Build history of the part. All positions in model axes, mm. A direction names the side the tool comes from. Round coordinates to 2 decimals unless told otherwise and drop trailing zeros. Loops run counter-clockwise (first coordinate to the right, second up) from the corner with the lowest first, then second, coordinate; pieces in that order, holes last. Notation, with made-up numbers: (-22.75, 24.25) -> (12.25, 24.25) arc R30 ccw to (12.25, 55.25) -> close; hole circle Ø9 at (47.25, 5). An arc over 180 degrees is marked (long way). Put each result on its own line as item: value. Start each with the question number.
Item 1: Cut at A-A, the plane x = 7.5. Count the separate pieces of the cut face and the enclosed holes in it, plus the area to 3 significant figures.
Item 2: Cut at D-D, the plane y = -10. List the corners of the cut face in (x, z), plus the area to 3 significant figures.
Item 3: Cut at C-C, the plane z = 26. List the corners of the cut face in (x, y).
Item 4: Pull direction Z, two halves, no side cores. Call faces 1 (the flat face through (15, -5, 27.5)), 2 (the flat face through (23, -23, 5)), 3 (the cylindrical face through (0.57, -39.4, 17.74)), 4 (the flat face through (3, -7.349, 29)): +Z half, -Z half, draft (parallel to the pull), parting line (faces both ways), or undercut.
Item 5: Flat gauge pins, fed straight in: pin 1 Ø5.5 at (x, y) = (22.5, -10) entering from +Z; pin 2 Ø3 at (x, y) = (7.5, -25) entering from -Z. Where does each tip first touch, or does it go through?
Item 6: Cut at B-B, the plane y = -5. List the corners of the cut face in (x, z).
Item 7: Drill centre lines: probe 1 along Y at (x, z) = (11, 28.5); probe 2 along Y at (x, z) = (22.5, 3.85); probe 3 along Z at (x, y) = (27.5, -5.5). Where is each one in solid material? Low to high. Write a range as [from, to].
Item 8: Tool access for faces 5 (the cylindrical face through (4.881, -12.008, 20.21)), 6 (the cylindrical face through (0.57, -0.6, 17.74)), 7 (the flat face through (15, -5, 30)): list every direction of +Z, -Z, +X, -X, +Y, -Y with a clear straight run to the whole face (end or side of a thin tool).
```python
from build123d import *

# Parameters (mm, degrees)
F0_W      = 30
F0_H      = 40
F1_DEPTH  = 35
F2_R      = 3.3
F3_DEPTH  = 30
F4_W      = 5
F4_H      = 2.5
F5_DEPTH  = 30.001
F6_R      = 1.65
F7_DEPTH  = 5.001
F8_R      = 1.65
F9_DEPTH  = 5.001
F10_R     = 1.65
F11_DEPTH = 5.001
F12_R     = 1.65
F13_DEPTH = 5.001
F14_R     = 2


with BuildPart() as f1:
    # F0 (on Top) → F1 (new body)
    with BuildSketch(Plane.XY):
        with Locations((15, -20)):
            Rectangle(F0_W, F0_H)
    extrude(amount=F1_DEPTH)

    # F2 (on face) → F3 (cut)
    with BuildSketch(Plane.XY.offset(35)):
        with Locations((7.5, -10)):
            Circle(F2_R)
        with Locations((22.5, -10)):
            Circle(F2_R)
        with Locations((7.5, -25)):
            Circle(F2_R)
        with Locations((22.5, -25)):
            Circle(F2_R)
    extrude(amount=-F3_DEPTH, mode=Mode.SUBTRACT)

    # F4 (on face) → F5 (cut, through all)
    with BuildSketch(Plane(origin=(0, 0, 0), x_dir=(0, -1, 0), z_dir=(-1, 0, 0))):
        with Locations((4.849052, 28.75)):
            Rectangle(F4_W, F4_H)
        with Locations((17.696945, 28.75)):
            Rectangle(F4_W, F4_H)
        with Locations((34.58895, 28.75)):
            Rectangle(F4_W, F4_H)
    extrude(amount=-F5_DEPTH, mode=Mode.SUBTRACT)

    # F6 (on face) → F7 (cut, through all)
    with BuildSketch(Plane.XY.offset(5)):
        with Locations((7.5, -10)):
            Circle(F6_R)
    extrude(amount=-F7_DEPTH, mode=Mode.SUBTRACT)

    # F8 (on face) → F9 (cut, through all)
    with BuildSketch(Plane.XY.offset(5)):
        with Locations((7.5, -25)):
            Circle(F8_R)
    extrude(amount=-F9_DEPTH, mode=Mode.SUBTRACT)

    # F10 (on face) → F11 (cut, through all)
    with BuildSketch(Plane.XY.offset(5)):
        with Locations((22.5, -25)):
            Circle(F10_R)
    extrude(amount=-F11_DEPTH, mode=Mode.SUBTRACT)

    # F12 (on face) → F13 (cut, through all)
    with BuildSketch(Plane.XY.offset(5)):
        with Locations((22.5, -10)):
            Circle(F12_R)
    extrude(amount=-F13_DEPTH, mode=Mode.SUBTRACT)

    # F14
    f14_edges = [f1.edges().sort_by_distance(p)[0] for p in [
        (0, 0, 17.5),
        (30, 0, 17.5),
        (30, -40, 17.5),
        (0, -40, 17.5),
    ]]
    fillet(f14_edges, radius=F14_R)


solid = f1.part
```
Reply:
1. separate pieces: 3
1. enclosed holes: 2
1. area: 935 mm^2
2. outline: (0, 0) -> (5.85, 0) -> (5.85, 5) -> (4.2, 5) -> (4.2, 35) -> (0, 35) -> close; (9.15, 0) -> (20.85, 0) -> (20.85, 5) -> (19.2, 5) -> (19.2, 35) -> (10.8, 35) -> (10.8, 5) -> (9.15, 5) -> close; (24.15, 0) -> (30, 0) -> (30, 35) -> (25.8, 35) -> (25.8, 5) -> (24.15, 5) -> close
2. area: 621 mm^2
3. outline: (0, -38) arc R2 ccw to (2, -40) -> (28, -40) arc R2 ccw to (30, -38) -> (30, -2) arc R2 ccw to (28, 0) -> (2, 0) arc R2 ccw to (0, -2) -> close; hole circle Ø6.6 at (7.5, -25); hole circle Ø6.6 at (7.5, -10); hole circle Ø6.6 at (22.5, -25); hole circle Ø6.6 at (22.5, -10)
4. face 1: undercut
4. face 2: +Z half
4. face 3: draft
4. face 4: undercut
5. pin 1: stops at z = 5
5. pin 2: passes through
6. outline: (0, 0) -> (30, 0) -> (30, 27.5) -> (0, 27.5) -> close; (0, 30) -> (30, 30) -> (30, 35) -> (0, 35) -> close
7. probe 1: y = [-40, -37.09], [-32.09, -20.2], [-15.2, -7.35], [-2.35, 0]
7. probe 2: y = [-40, -26.65], [-23.35, -11.65], [-8.35, 0]
7. probe 3: z = [0, 27.5], [30, 35]
8. face 5: +Z
8. face 6: +Z, -Z, -X, +Y
8. face 7: +X, -X
